Autodesk Inventor part; units mm, degrees
ref_plane "YZ Plane" through (0, 0, 0) normal (1, 0, 0) x (0, 1, 0)
ref_plane "XZ Plane" through (0, 0, 0) normal (0, 1, 0) x (-1, 0, 0)
ref_plane "XY Plane" through (0, 0, 0) normal (0, 0, 1) x (1, 0, 0)
sketch "Sketch1" plane through (0, 0, 0) normal (0, 1, 0) x (-1, 0, 0)
  circle A0 centre (0, 0) radius 50
  dimension "d0" = 100
extrude "Extrusion1" add sketch "Sketch1" along normal blind 3
sketch "Sketch2" plane through (0, 3, 0) normal (0, 1, 0) x (1, 0, 0)
  line L0 (-5, -41) -> (5, -41)
  line L1 (5, -41) -> (5, -38)
  line L2 (5, -38) -> (-5, -38)
  line L3 (-5, -38) -> (-5, -41)
  line L4 (-5, 38) -> (5, 38)
  line L5 (5, 38) -> (5, 41)
  line L6 (5, 41) -> (-5, 41)
  line L7 (-5, 41) -> (-5, 38)
  point P0 (0, 0)
  dimension "d3" = 10
  dimension "d4" = 3
  dimension "d5" = 5
  dimension "d6" = 38
  dimension "d7" = 10
  dimension "d8" = 3
  dimension "d9" = 5
  dimension "d10" = 38
extrude "Extrusion2" cut sketch "Sketch2" against normal blind 3
properties part number "face"
Check sheet for the modelled part. Datum: model origin and axes. Units: mm. A direction names the side the tool comes from. Round coordinates to 2 decimals unless told otherwise and drop trailing zeros. Loops run counter-clockwise (first coordinate to the right, second up) from the corner with the lowest first, then second, coordinate; pieces in that order, holes last. Notation, with made-up numbers: (84, -1) -> (110, -1) arc R15 cw to (110, 24) -> close; hole circle Ø7 at (18, 36). An arc over 180 degrees is marked (long way). Answer in a Markdown table with one row per item.
Q1. Release check for a two-part mould opening along Z. For faces 1 (the face through (-47.69, 1.48, -15.02)), 2 (the face through (1, 0, 1)), 3 (the face through (5, 2, 40)) record: released by +Z, released by -Z, zero draft, split by the parting line, or undercut.
Data:
| item | result |
|---|---|
| face 1 | split by the parting line |
| face 2 | zero draft |
| face 3 | undercut |
Q2. Thickness scan on L1, parallel to Z at x = 3, y = 0.75; L2, parallel to Z at x = 2, y = 1.7; L3, parallel to X at y = 0.7, z = 1.5. Record the ranges inside material, lowest first.
Data:
| item | result |
|---|---|
| L1 | z = -49.91 to -41, -38 to 38, 41 to 49.91 |
| L2 | z = -49.96 to -41, -38 to 38, 41 to 49.96 |
| L3 | x = -49.98 to 49.98 |
Q3. Sectioned sample at C-C on z = 30. Enter the section's corners in (x, y).
Data:
| item | result |
|---|---|
| outline | (-40, 0) -> (40, 0) -> (40, 3) -> (-40, 3) -> close |
Q4. Sectioned sample at D-D on x = 38. Enter the section's corners in (y, z).
Data:
| item | result |
|---|---|
| outline | (0, -32.5) -> (3, -32.5) -> (3, 32.5) -> (0, 32.5) -> close |
Q5. Sectioned sample at B-B on x = 0. Enter the section's corners in (y, z), then the cut area to 3 significant figures.
Data:
| item | result |
|---|---|
| outline | (0, -50) -> (3, -50) -> (3, -41) -> (0, -41) -> close; (0, -38) -> (3, -38) -> (3, 38) -> (0, 38) -> close; (0, 41) -> (3, 41) -> (3, 50) -> (0, 50) -> close |
| area | 282 mm^2 |
Q6. Set-up check for faces 4 (the face through (0, 2, -38)), 5 (the face through (1, 3, 1)): record each of +Z, -Z, +X, -X, +Y, -Y from which the full face is reachable in a straight line by a thin tool's end or side.
Data:
| item | result |
|---|---|
| face 4 | +Y, -Y |
| face 5 | +Z, -Z, +X, -X, +Y |
Q7. Go/stop test with flat-tipped pins: P1, Ø1, axis at y = 2.5, z = 16.5, coming from the -X side; P2, Ø1.5, axis at x = 18.5, y = 1, coming from the +Z side; P3, Ø1, axis at x = 2, z = -18, coming from the -Y side; P4, Ø0.9, axis at x = -0.5, y = 1.5, coming from the +Z side. Record where each tip stops, or that it passes through.
Data:
| item | result |
|---|---|
| P1 | stops at x = -47.37 |
| P2 | stops at z = 46.74 |
| P3 | stops at y = 0 |
| P4 | stops at z = 50 |
Q8. Sectioned sample at A-A on y = 0.75. Enter the section's corners in (x, z).
Data:
| item | result |
|---|---|
| outline | circle Ø100 at (0, 0); hole (-5, -41) -> (5, -41) -> (5, -38) -> (-5, -38) -> close; hole (-5, 38) -> (5, 38) -> (5, 41) -> (-5, 41) -> close |
